Source: CAD feature listing. Evaluate the final solid. Frame: model axes, mm. Face numbers are marked on the shaded views. A direction names the side the tool comes from. Give positions to 0.01 mm unless a question says otherwise; leave off trailing zeros. Write each loop counter-clockwise with the first axis right and the second up, starting at its lowest first coordinate (ties: lowest second). Pieces come first, ordered by that corner, then holes. Notation, with made-up numbers: M 59,89 L 92,89 A20 ccw 92,116 Z; hole C -20,19 d7. An arc over 180 degrees is marked long. Use CSV: the item, a comma, the result in double quotes. Start each with the question number.
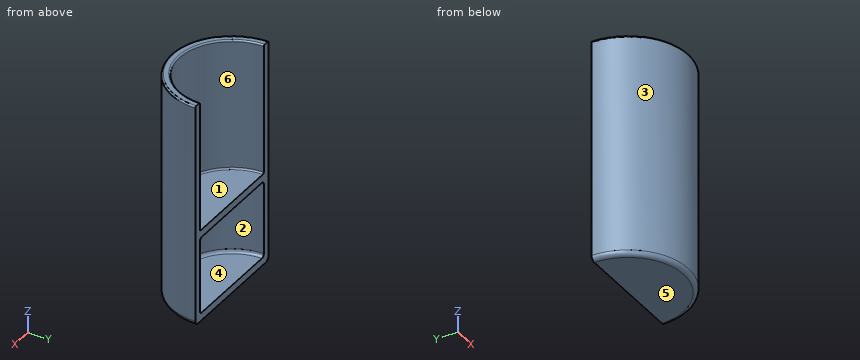
from build123d import *

# Parameters (mm, degrees)
F1_ANGLE = 180


with BuildPart() as f1:
    # F0 (on Front) → F1 (revolve)
    with BuildSketch(Plane.XZ):
        with BuildLine():
            ThreePointArc((39, 42.814617), (38.707107, 43.521724), (38, 43.814617))
            Line((38, 43.814617), (35, 43.814617))
            ThreePointArc((35, 43.814617), (34.292893, 43.521724), (34, 42.814617))
            Line((34, 42.814617), (34, -40.185383))
            ThreePointArc((34, -40.185383), (33.707107, -40.89249), (33, -41.185383))
            Line((33, -41.185383), (0, -41.185383))
            Line((0, -41.185383), (0, -46.185383))
            Line((0, -46.185383), (32, -46.185383))
            ThreePointArc((32, -46.185383), (33.414214, -46.77117), (34, -48.185383))
            Line((34, -48.185383), (34, -94.185383))
            ThreePointArc((34, -94.185383), (33.414214, -95.599597), (32, -96.185383))
            Line((32, -96.185383), (0, -96.185383))
            Line((0, -96.185383), (0, -101.185383))
            Line((0, -101.185383), (36, -101.185383))
            ThreePointArc((36, -101.185383), (38.12132, -100.306703), (39, -98.185383))
            Line((39, -98.185383), (39, 42.814617))
        make_face()
    revolve(axis=Axis((0, 0, -39.313186), (0, 0, -1)), revolution_arc=F1_ANGLE)


solid = f1.part
Item 1: Set-up query: the marked faces 4, 5 and 6. Return all of +Z, -Z, +X, -X, +Y, -Y with unobstructed straight access to the full face (end or side cutting, diameter ignored); none if empty.
Item 2: Section A-A (x = 0). Return the cut outline in (y, z).
Item 3: Section B-B (z = -78). Return the cut outline in (x, y).
Item 4: Pull-direction query (Z, two-part tool) for the marked faces 1, 2 and 3; classes: released by +Z, released by -Z, zero draft, split by the parting line, or undercut.
Item 5: Contact query for flat-ended pins moving along their axis: pin 1 Ø6 at (y, z) = (-29.5, 4) entering from -X; pin 2 Ø6 at (y, z) = (-29.5, -44.5) entering from +X; pin 3 Ø6 at (x, z) = (-1.5, -81.5) entering from +Y. Output: stop coordinate, or through.
Item 6: Material intervals for probe 1 along Z at (x, y) = (-17.5, -19); probe 2 along X at (y, z) = (-22, -2); probe 3 along X at (y, z) = (-29, -69), sorted ascending.
Output values:
1,face 4,"+Y"
1,face 5,"-Z, +X, -X, +Y, -Y"
1,face 6,"+Z, +Y"
2,outline,"M -39,-98.19 A3 ccw -36,-101.19 L 0,-101.19 L 0,-96.19 L -32,-96.19 A2 cw -34,-94.19 L -34,-48.19 A2 cw -32,-46.19 L 0,-46.19 L 0,-41.19 L -33,-41.19 A1 cw -34,-40.19 L -34,42.81 A1 ccw -35,43.81 L -38,43.81 A1 ccw -39,42.81 Z"
3,outline,"M -39,0 A39 ccw 39,0 L 34,0 A34 cw -34,0 Z"
4,face 1,"released by +Z"
4,face 2,"undercut"
4,face 3,"zero draft"
5,pin 1,"stops at x = -28.61"
5,pin 2,"stops at x = 28.61"
5,pin 3,"stops at y = -33.7"
6,probe 1,"z = -101.19 to -96.19, -46.19 to -41.19"
6,probe 2,"x = -32.2 to -25.92, 25.92 to 32.2"
6,probe 3,"x = -26.08 to -17.75, 17.75 to 26.08"
